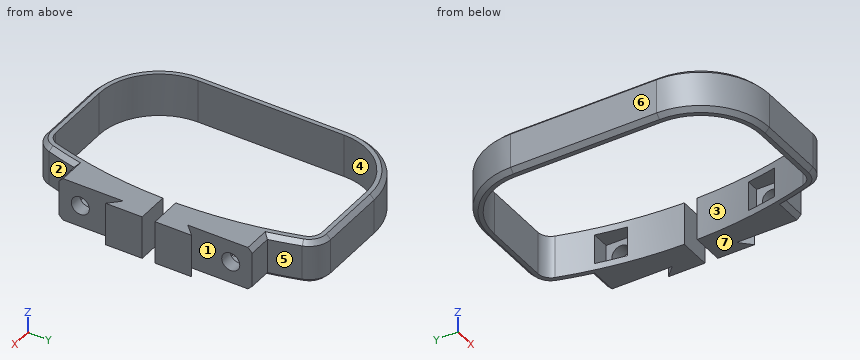
```python
from build123d import *

# Parameters (mm, degrees)
SALIENTE_EXTRUIR1_DEPTH = 5
SALIENTE_EXTRUIR2_DEPTH = 10
CORTAR_EXTRUIR1_DEPTH   = 11
CROQUIS4_W              = 15
CROQUIS4_H              = 3
CORTAR_EXTRUIR2_DEPTH   = 11
CORTAR_EXTRUIR3_REACH   = 46
CROQUIS6_R              = 2.1
CORTAR_EXTRUIR4_REACH   = 49
CORTAR_EXTRUIR4_START   = -3
CROQUIS7_W              = 6.9
CROQUIS7_H              = 6.9
CHAFL_N1_SIZE           = 1


with BuildPart() as part:
    # Croquis1 → Saliente-Extruir1 (new body, symmetric)
    with BuildSketch(Plane.XY):
        with BuildLine():
            Line((-20.5, -17), (-20.5, 17))
            ThreePointArc((-20.5, 17), (-15.813708499, 28.313708499), (-4.5, 33))
            Line((-4.5, 33), (11.370878105, 33))
            ThreePointArc((11.370878105, 33), (14.352782292, 32.013508119), (16.15803677, 29.443298969))
            ThreePointArc((16.15803677, 29.443298969), (20.5, 0), (16.15803677, -29.443298969))
            ThreePointArc((16.15803677, -29.443298969), (14.352782292, -32.013508119), (11.370878105, -33))
            Line((11.370878105, -33), (-4.5, -33))
            ThreePointArc((-4.5, -33), (-15.813708499, -28.313708499), (-20.5, -17))
        make_face()
        with BuildLine():
            Line((-4.5, 31), (11.370878105, 31))
            ThreePointArc((11.370878105, 31), (13.160020617, 30.408104872), (14.243173304, 28.865979381))
            ThreePointArc((14.243173304, 28.865979381), (18.5, 0), (14.243173304, -28.865979381))
            ThreePointArc((14.243173304, -28.865979381), (13.160020617, -30.408104872), (11.370878105, -31))
            Line((11.370878105, -31), (-4.5, -31))
            ThreePointArc((-4.5, -31), (-14.399494937, -26.899494937), (-18.5, -17))
            Line((-18.5, -17), (-18.5, 17))
            ThreePointArc((-18.5, 17), (-14.399494937, 26.899494937), (-4.5, 31))
        make_face(mode=Mode.SUBTRACT)
    extrude(amount=SALIENTE_EXTRUIR1_DEPTH, both=True)

    # Croquis2 → Saliente-Extruir2 (add, through all)
    with BuildSketch(Plane.XY.offset(5)):
        Polygon((18.5, 22.5), (17.987436393, 22.5), (20.5, 0), (17.987436393, -22.5), (18.5, -22.5), (28.5, -22.5), (28.5, 22.5), align=None)
    extrude(amount=-SALIENTE_EXTRUIR2_DEPTH)

    # Croquis3 → Cortar-Extruir1 (cut, through all)
    with BuildSketch(Plane.XY.offset(5)):
        Polygon((23.5, 22.5), (23.5, 7.5), (26, 10), (26, -10), (23.5, -7.5), (23.5, -22.5), (28.5, -22.5), (28.5, 22.5), align=None)
    extrude(amount=-CORTAR_EXTRUIR1_DEPTH, mode=Mode.SUBTRACT)

    # Croquis4 → Cortar-Extruir2 (cut, through all)
    with BuildSketch(Plane.XY.offset(5)):
        with Locations((18.5, 0)):
            Rectangle(CROQUIS4_W, CROQUIS4_H)
    extrude(amount=-CORTAR_EXTRUIR2_DEPTH, mode=Mode.SUBTRACT)

    # Croquis6 → Cortar-Extruir3 (cut, up to next)
    with BuildSketch(Plane(origin=(23.5, 0, 0), x_dir=(0, 0, -1), z_dir=(1, 0, 0)), mode=Mode.PRIVATE) as cortar_extruir3_sk1:
        with Locations((0, 17.5)):
            Circle(CROQUIS6_R)
    cortar_extruir3_tool1 = extrude(cortar_extruir3_sk1.sketch, amount=-CORTAR_EXTRUIR3_REACH, mode=Mode.PRIVATE) & part.part
    add(cortar_extruir3_tool1.solids().sort_by_distance((23.5, 17.5, 0))[0], mode=Mode.SUBTRACT)
    # Croquis6 → Cortar-Extruir3 (cut, up to next)
    with BuildSketch(Plane(origin=(23.5, 0, 0), x_dir=(0, 0, -1), z_dir=(1, 0, 0)), mode=Mode.PRIVATE) as cortar_extruir3_sk2:
        with Locations((0, -17.5)):
            Circle(CROQUIS6_R)
    cortar_extruir3_tool2 = extrude(cortar_extruir3_sk2.sketch, amount=-CORTAR_EXTRUIR3_REACH, mode=Mode.PRIVATE) & part.part
    add(cortar_extruir3_tool2.solids().sort_by_distance((23.5, -17.5, 0))[0], mode=Mode.SUBTRACT)

    # Croquis7 → Cortar-Extruir4 (cut, up to next)
    with BuildSketch(Plane(origin=(23.5, 0, 0), x_dir=(0, 0, -1), z_dir=(1, 0, 0)).offset(CORTAR_EXTRUIR4_START), mode=Mode.PRIVATE) as cortar_extruir4_sk1:
        with Locations((0, 17.5)):
            Rectangle(CROQUIS7_W, CROQUIS7_H)
    cortar_extruir4_tool1 = extrude(cortar_extruir4_sk1.sketch, amount=-CORTAR_EXTRUIR4_REACH, mode=Mode.PRIVATE) & part.part
    add(cortar_extruir4_tool1.solids().sort_by_distance((20.5, 17.5, 0))[0], mode=Mode.SUBTRACT)
    # Croquis7 → Cortar-Extruir4 (cut, up to next)
    with BuildSketch(Plane(origin=(23.5, 0, 0), x_dir=(0, 0, -1), z_dir=(1, 0, 0)).offset(CORTAR_EXTRUIR4_START), mode=Mode.PRIVATE) as cortar_extruir4_sk2:
        with Locations((0, -17.5)):
            Rectangle(CROQUIS7_W, CROQUIS7_H)
    cortar_extruir4_tool2 = extrude(cortar_extruir4_sk2.sketch, amount=-CORTAR_EXTRUIR4_REACH, mode=Mode.PRIVATE) & part.part
    add(cortar_extruir4_tool2.solids().sort_by_distance((20.5, -17.5, 0))[0], mode=Mode.SUBTRACT)

    # Chaflán1
    chafl_n1_edges = [part.edges().sort_by_distance(p)[0] for p in [
        (3.435439053, -33, -5),
        (-15.813708499, -28.313708499, -5),
        (-20.5, 0, -5),
        (-15.813708499, 28.313708499, -5),
        (-15.813708499, -28.313708499, 5),
        (3.435439053, -33, 5),
        (14.352782292, -32.013508119, 5),
        (17.133851934, -25.987751975, 5),
        (14.352782292, 32.013508119, 5),
        (3.435439053, 33, 5),
        (-15.813708499, 28.313708499, 5),
        (17.133851934, 25.987751975, -5),
        (17.133851934, 25.987751975, 5),
        (20.743718196, -22.5, -5),
        (20.743718196, -22.5, 5),
        (20.743718196, 22.5, 5),
        (20.743718196, 22.5, -5),
        (3.435439053, 33, -5),
        (-20.5, 0, 5),
        (14.352782292, 32.013508119, -5),
        (17.133851934, -25.987751975, -5),
        (14.352782292, -32.013508119, -5),
    ]]
    chamfer(chafl_n1_edges, length=CHAFL_N1_SIZE)


solid = part.part
```
Read the model definition and answer for the solid it produces. Units are mm, in the model's axes. Face numbers are marked on the shaded views. A direction names the side the tool comes from. Coordinates: 2 decimals unless noted, no trailing zeros. Write each loop counter-clockwise with the first axis right and the second up, starting at its lowest first coordinate (ties: lowest second). Pieces come first, ordered by that corner, then holes. Notation, with made-up numbers: (71.25, -31) -> (115.25, -31) arc R25 ccw to (115.25, -1) -> close; hole circle Ø1 at (67, -32.75). An arc over 180 degrees is marked (long way). Answer as a JSON object with one key per item and string values.
Q1. The part is cut by section C-C on z = 0. Give the number of separate pieces and of enclosed holes in the cut face, then the cut area to 3 significant figures.
The answers:
{"separate pieces": "3", "enclosed holes": "0", "area": "484 mm2"}
Q2. The part is cut by section B-B on y = 3. Give the vertices of the cut face in (x, z).
The answers:
{"outline": "(-20.5, -4) -> (-19.5, -5) -> (-18.5, -5) -> (-18.5, 5) -> (-19.5, 5) -> (-20.5, 4) -> close; (18.45, -5) -> (26, -5) -> (26, 5) -> (18.45, 5) -> close"}
Q3. Consider line 1 (Y direction, x = 22.1, z = 0); line 2 (Y direction, x = 5.5, z = -3.5); line 3 (X direction, y = 15.5, z = 2.25). Determine where each line is inside the solid, lowest interval first. Write a range as [from, to].
The answers:
{"line 1": "y = [-22.5, -19.6], [-15.4, -1.5], [1.5, 15.4], [19.6, 22.5]", "line 2": "y = [-33, -31], [31, 33]", "line 3": "x = [-20.5, -18.5], [20.5, 23.5]"}
Q4. Determine the mould class of the marked faces 4, 5, 6 and 7 for opening direction X: pulls with the +X half, pulls with the -X half, needs draft (parallel to the pull), parting line crosses it, or undercut.
The answers:
{"face 4": "undercut", "face 5": "pulls with the +X half", "face 6": "pulls with the -X half", "face 7": "needs draft"}
Q5. A tool of negligible diameter and unlimited length cuts with its end or side. For the marked faces 1, 2 and 3, from which of +Z, -Z, +X, -X, +Y, -Y can it reach the whole face along a straight path? Write none if from no direction.
The answers:
{"face 1": "+Z, -Z, +Y", "face 2": "+Z, -Z, +X, -Y", "face 3": "+Z, -Z"}
Q6. The part is cut by section A-A on x = 19.5. Give the vertices of the cut face in (y, z), then the cut area to 3 significant figures.
The answers:
{"outline": "(-22.5, -4) -> (-21.5, -5) -> (-1.5, -5) -> (-1.5, 5) -> (-21.5, 5) -> (-22.5, 4) -> close; (1.5, -5) -> (21.5, -5) -> (22.5, -4) -> (22.5, 4) -> (21.5, 5) -> (1.5, 5) -> close; hole (-20.95, -3.45) -> (-14.05, -3.45) -> (-14.05, 3.45) -> (-20.95, 3.45) -> close; hole (14.05, -3.45) -> (20.95, -3.45) -> (20.95, 3.45) -> (14.05, 3.45) -> close", "area": "323 mm2"}
Q7. Flat-ended cylindrical pins translate along their axes: pin 1 Ø1 at (x, z) = (-9, 1) entering from +Y; pin 2 Ø5 at (y, z) = (-17, 2) entering from +X; pin 3 Ø1.3 at (x, z) = (19, -1.5) entering from -Y. Find the tip coordinate at first contact, or state that the pin passes through.
The answers:
{"pin 1": "stops at y = 32.49", "pin 2": "stops at x = 23.5", "pin 3": "stops at y = -22.5"}
